The drawing under review shows one solid part. Ordinate dimensions are in mm from its lowest x, y, z. Round coordinates to 2 decimals unless told otherwise and drop trailing zeros. Order: outer loops, then holes, each group sorted by start corner. A loop starts at its lowest first (then second) coordinate and runs counter-clockwise, first axis right, second up. Notation, with made-up numbers: M -36.75,56 L 2.25,56 A20 ccw 2.25,83 Z; hole C -16,6 d4. An arc over 180 degrees is marked long. Answer as a JSON object with one key per item and string values.
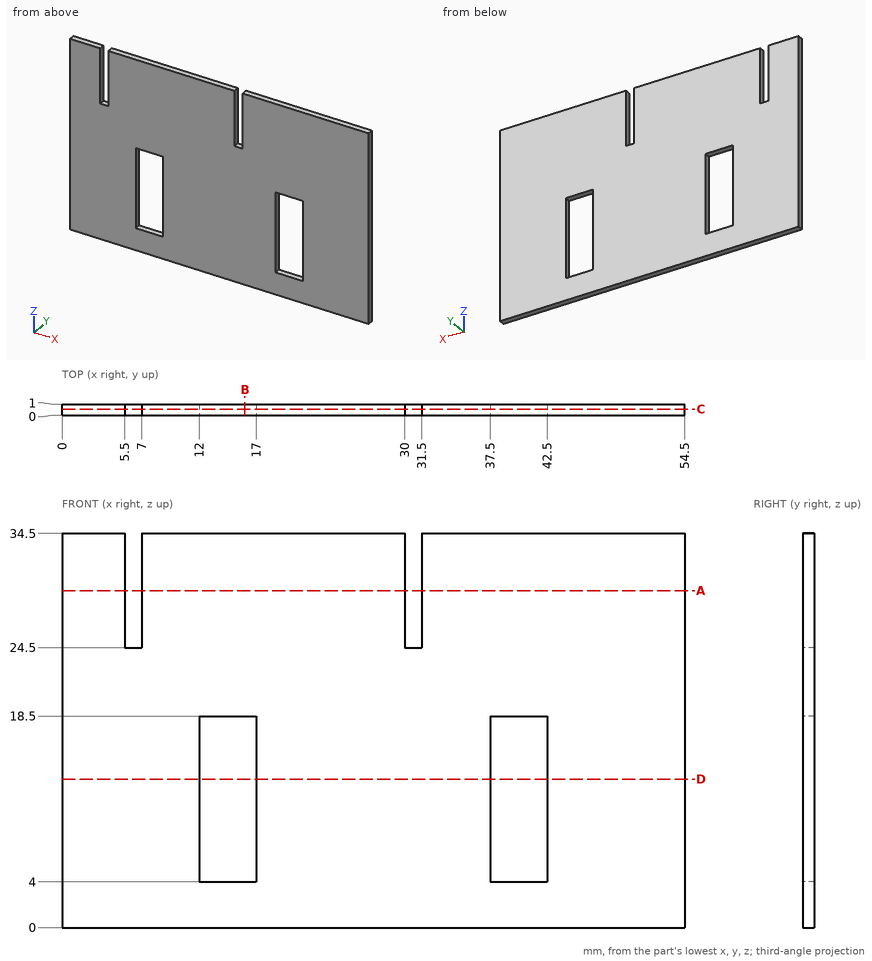
1) For L1, parallel to X at y = 0.5, z = 32.5; L2, parallel to X at y = 0.75, z = 15; L3, parallel to Z at x = 6.5, y = 0.1, list the stretches that pass through material, from the lowest coordinate up.
Geometry check:
{"L1": "x = 0 to 5.5, 7 to 30, 31.5 to 54.5", "L2": "x = 0 to 12, 17 to 37.5, 42.5 to 54.5", "L3": "z = 0 to 24.5"}
2) Add section D-D on z = 13. State the section outline as (x, y) points.
Geometry check:
{"outline": "M 0,0 L 12,0 L 12,1 L 0,1 Z; M 17,0 L 37.5,0 L 37.5,1 L 17,1 Z; M 42.5,0 L 54.5,0 L 54.5,1 L 42.5,1 Z"}
3) Add section B-B on x = 16. State the section outline as (y, z) points.
Geometry check:
{"outline": "M 0,0 L 1,0 L 1,4 L 0,4 Z; M 0,18.5 L 1,18.5 L 1,34.5 L 0,34.5 Z"}
4) Add section A-A on z = 29.5. State the section outline as (x, y) points, and give its area (3 significant figures).
Geometry check:
{"outline": "M 0,0 L 5.5,0 L 5.5,1 L 0,1 Z; M 7,0 L 30,0 L 30,1 L 7,1 Z; M 31.5,0 L 54.5,0 L 54.5,1 L 31.5,1 Z", "area": "51.5 mm²"}
5) Add section C-C on y = 0.55. State the section outline as (x, z) points, and give its area (3 significant figures).
Geometry check:
{"outline": "M 0,0 L 54.5,0 L 54.5,34.5 L 31.5,34.5 L 31.5,24.5 L 30,24.5 L 30,34.5 L 7,34.5 L 7,24.5 L 5.5,24.5 L 5.5,34.5 L 0,34.5 Z; hole M 12,4 L 17,4 L 17,18.5 L 12,18.5 Z; hole M 37.5,4 L 42.5,4 L 42.5,18.5 L 37.5,18.5 Z", "area": "1,710 mm²"}
